```python
from build123d import *

# Parameters (mm, degrees)
EXTRUDE_1_DEPTH     = 1500
SKETCH_2_R          = 5
CUT_EXTRUDE_1_DEPTH = 46
SKETCH_3_R          = 5
CUT_EXTRUDE_2_DEPTH = 46


with BuildPart() as part:
    # Эскиз1 → Вытянуть-Тонкостенный1 (new body)
    with BuildSketch(Plane(origin=(0, 0, 0), x_dir=(0, 0, -1), z_dir=(1, 0, 0))):
        Polygon((45, 0), (0, 0), (0, 45), (4, 45), (4, 4), (45, 4), align=None)
    extrude(amount=EXTRUDE_1_DEPTH)

    # Эскиз2 → Вырез-Вытянуть1 (cut, through all)
    with BuildSketch(Plane.XY):
        with Locations((30, 25)):
            Circle(SKETCH_2_R)
        with Locations((90, 25)):
            Circle(SKETCH_2_R)
        with Locations((150, 25)):
            Circle(SKETCH_2_R)
        with Locations((210, 25)):
            Circle(SKETCH_2_R)
        with Locations((270, 25)):
            Circle(SKETCH_2_R)
        with Locations((330, 25)):
            Circle(SKETCH_2_R)
        with Locations((390, 25)):
            Circle(SKETCH_2_R)
        with Locations((450, 25)):
            Circle(SKETCH_2_R)
        with Locations((510, 25)):
            Circle(SKETCH_2_R)
        with Locations((570, 25)):
            Circle(SKETCH_2_R)
        with Locations((630, 25)):
            Circle(SKETCH_2_R)
        with Locations((690, 25)):
            Circle(SKETCH_2_R)
        with Locations((750, 25)):
            Circle(SKETCH_2_R)
        with Locations((810, 25)):
            Circle(SKETCH_2_R)
        with Locations((870, 25)):
            Circle(SKETCH_2_R)
        with Locations((930, 25)):
            Circle(SKETCH_2_R)
        with Locations((990, 25)):
            Circle(SKETCH_2_R)
        with Locations((1050, 25)):
            Circle(SKETCH_2_R)
        with Locations((1110, 25)):
            Circle(SKETCH_2_R)
        with Locations((1170, 25)):
            Circle(SKETCH_2_R)
        with Locations((1230, 25)):
            Circle(SKETCH_2_R)
        with Locations((1290, 25)):
            Circle(SKETCH_2_R)
        with Locations((1350, 25)):
            Circle(SKETCH_2_R)
        with Locations((1410, 25)):
            Circle(SKETCH_2_R)
        with Locations((1470, 25)):
            Circle(SKETCH_2_R)
    extrude(amount=-CUT_EXTRUDE_1_DEPTH, mode=Mode.SUBTRACT)

    # Эскиз3 → Вырез-Вытянуть2 (cut, through all)
    with BuildSketch(Plane.XZ):
        with Locations((30, -25)):
            Circle(SKETCH_3_R)
        with Locations((90, -25)):
            Circle(SKETCH_3_R)
        with Locations((150, -25)):
            Circle(SKETCH_3_R)
        with Locations((210, -25)):
            Circle(SKETCH_3_R)
        with Locations((270, -25)):
            Circle(SKETCH_3_R)
        with Locations((330, -25)):
            Circle(SKETCH_3_R)
        with Locations((390, -25)):
            Circle(SKETCH_3_R)
        with Locations((450, -25)):
            Circle(SKETCH_3_R)
        with Locations((510, -25)):
            Circle(SKETCH_3_R)
        with Locations((570, -25)):
            Circle(SKETCH_3_R)
        with Locations((630, -25)):
            Circle(SKETCH_3_R)
        with Locations((690, -25)):
            Circle(SKETCH_3_R)
        with Locations((750, -25)):
            Circle(SKETCH_3_R)
        with Locations((810, -25)):
            Circle(SKETCH_3_R)
        with Locations((870, -25)):
            Circle(SKETCH_3_R)
        with Locations((930, -25)):
            Circle(SKETCH_3_R)
        with Locations((990, -25)):
            Circle(SKETCH_3_R)
        with Locations((1050, -25)):
            Circle(SKETCH_3_R)
        with Locations((1110, -25)):
            Circle(SKETCH_3_R)
        with Locations((1170, -25)):
            Circle(SKETCH_3_R)
        with Locations((1230, -25)):
            Circle(SKETCH_3_R)
        with Locations((1290, -25)):
            Circle(SKETCH_3_R)
        with Locations((1350, -25)):
            Circle(SKETCH_3_R)
        with Locations((1410, -25)):
            Circle(SKETCH_3_R)
        with Locations((1470, -25)):
            Circle(SKETCH_3_R)
    extrude(amount=-CUT_EXTRUDE_2_DEPTH, mode=Mode.SUBTRACT)


solid = part.part
```
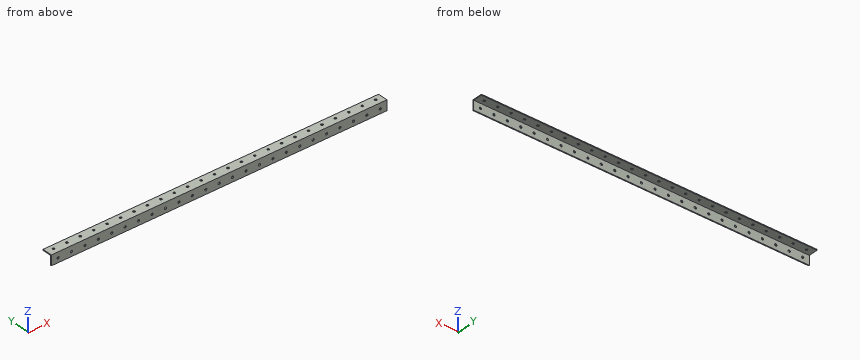
Input: part model. Units: mm. Frame: model coordinates. Give positions to 0.01 mm unless a question says otherwise; leave off trailing zeros. Loops run counter-clockwise (first coordinate to the right, second up) from the corner with the lowest first, then second, coordinate; pieces in that order, holes last.
1) Section query B-B on z = -12.5. Return the cut outline in (x, y), and give its area (3 significant figures).
A:
outline: (0, 0) - (1500, 0) - (1500, 4) - (0, 4) - close
area: 6,000 mm2
2) Section query A-A on y = 38. Return the cut outline in (x, z).
A:
outline: (0, -4) - (1500, -4) - (1500, 0) - (0, 0) - close
3) Section query C-C on x = 349. Return the cut outline in (y, z).
A:
outline: (0, -45) - (4, -45) - (4, -4) - (45, -4) - (45, 0) - (0, 0) - close
4) Line query: L1, parallel to Z at x = 690, y = 0.95; L2, parallel to Y at x = 30, z = -1.1; L3, parallel to Y at x = 387, z = -43. Output: solid intervals per line, ascending.
A:
L1: z = -45 to -30, -20 to 0
L2: y = 0 to 20, 30 to 45
L3: y = 0 to 4
5) Contact query for flat-ended pins moving along their axis: pin 1 (11.5 mm diameter, centred on x = 270, y = 25, fed in from -Z); pin 2 (1 mm diameter, centred on x = 355.5, z = -32.5, fed in from +Y). Output: stop coordinate, or through.
A:
pin 1: stops at z = -4
pin 2: stops at y = 4
